Check sheet for the modelled part. Datum: model origin and axes. Units: mm. Coordinates: 2 decimals unless noted, no trailing zeros. Write each loop counter-clockwise with the first axis right and the second up, starting at its lowest first coordinate (ties: lowest second). Pieces come first, ordered by that corner, then holes. Notation, with made-up numbers: (-20.5, 35.25) - (-12.5, 35.25) arc R16 cw to (-12.5, 64.25) - close; hole circle Ø1 at (69.25, 59.5). An arc over 180 degrees is marked (long way). Use one line per item in the form item = value. Start each with the question number.
1. Cross-section at B-B on z = 1.25. Record the boundary of the cut face in (x, y), then the cut area to 3 significant figures.
2. Cross-section at A-A on x = -47. Record the boundary of the cut face in (y, z), then the cut area to 3 significant figures.
3. Scan lines: line 1 along X through (y, z) = (275.75, 1.6); line 2 along X through (y, z) = (280.75, 0.7); line 3 along X through (y, z) = (269, 0.65). Record each from-to range of solid material in increasing order.
Autodesk Inventor part; units mm, degrees
ref_plane "YZ Plane" through (0, 0, 0) normal (1, 0, 0) x (0, 1, 0)
ref_plane "XZ Plane" through (0, 0, 0) normal (0, 1, 0) x (-1, 0, 0)
ref_plane "XY Plane" through (0, 0, 0) normal (0, 0, 1) x (1, 0, 0)
sketch "Sketch1" plane through (0, 0, 0) normal (0, 0, 1) x (1, 0, 0)
  arc A0 (-89.3851, 275.0837) -> (-93.3851, 275.0837) centre (-91.3851, 275.0837) ccw
  line L0 (-89.3851, 275.0837) -> (-89.3851, 230.0837)
  arc A1 (-93.3851, 230.0837) -> (-89.3851, 230.0837) centre (-91.3851, 230.0837) ccw
  line L1 (-93.3851, 230.0837) -> (-93.3851, 275.0837)
  arc A2 (-44.3851, 275.0837) -> (-48.3851, 275.0837) centre (-46.3851, 275.0837) ccw
  line L2 (-44.3851, 275.0837) -> (-44.3851, 230.0837)
  arc A3 (-48.3851, 230.0837) -> (-44.3851, 230.0837) centre (-46.3851, 230.0837) ccw
  line L3 (-48.3851, 230.0837) -> (-48.3851, 275.0837)
  circle A4 centre (-6.132, -79.3472) radius 1.25
  circle A5 centre (-145.3842, 185.8247) radius 1.5
  circle A6 centre (-153.8932, -1.3222) radius 1.5
  circle A7 centre (-145.3842, -79.3472) radius 1.5
  circle A8 centre (-129.8902, 6.8528) radius 1.5
  circle A9 centre (-116.3012, -71.1722) radius 1.5
  circle A10 centre (-129.8902, 272.0247) radius 1.5
  circle A11 centre (-129.8902, 185.8247) radius 1.5
  circle A12 centre (-116.3012, 263.8497) radius 1.5
  circle A13 centre (17.871, -71.1722) radius 1.5
  circle A14 centre (-6.132, 6.8528) radius 1.5
  circle A15 centre (-19.721, -1.3222) radius 1.5
  circle A16 centre (17.871, 263.8497) radius 1.5
  circle A17 centre (9.362, 272.0247) radius 1.5
  circle A18 centre (9.362, 185.8247) radius 1.5
  circle A19 centre (-19.721, 193.9997) radius 1.5
  circle A20 centre (-19.721, 263.8497) radius 1.5
  circle A21 centre (-6.132, 185.8247) radius 1.5
  circle A22 centre (-6.132, 272.0247) radius 1.5
  circle A23 centre (17.871, 193.9997) radius 1.5
  circle A24 centre (-19.721, -71.1722) radius 1.5
  circle A25 centre (9.362, -79.3472) radius 1.5
  circle A26 centre (9.362, 6.8528) radius 1.5
  circle A27 centre (17.871, -1.3222) radius 1.5
  circle A28 centre (-116.3012, 193.9997) radius 1.5
  circle A29 centre (-153.8932, 193.9997) radius 1.5
  circle A30 centre (-153.8932, 263.8497) radius 1.5
  circle A31 centre (-145.3842, 6.8528) radius 1.5
  circle A32 centre (-129.8902, -79.3472) radius 1.5
  circle A33 centre (-153.8932, -71.1722) radius 1.5
  circle A34 centre (-116.3012, -1.3222) radius 1.5
  circle A35 centre (-145.3842, 272.0247) radius 1.5
  arc A36 (81.2372, 206.8201) -> (56.4499, 266.1206) centre (-44.5185, 189.0856) ccw
  ellipse E0 centre (-68.0111, 96.3387) end of major axis (-68.0111, -141.4053) minor radius 177.8 (56.4499, 266.1206) -> (-192.4721, 266.1206) ccw
  arc A37 (-192.4721, 266.1206) -> (-217.2594, 206.8201) centre (-91.5037, 189.0856) ccw
  arc A38 (-217.2594, 206.8201) -> (-217.2594, -14.1426) centre (566.1677, 96.3387) ccw
  arc A39 (-217.2594, -14.1426) -> (-192.4721, -73.4431) centre (-91.5037, 3.5918) ccw
  ellipse E1 centre (-68.0111, 96.3387) end of major axis (-68.0111, -141.4053) minor radius 177.8 (-192.4721, -73.4431) -> (56.4499, -73.4431) ccw
  arc A40 (56.4499, -73.4431) -> (81.2372, -14.1426) centre (-44.5185, 3.5918) ccw
  arc A41 (81.2372, -14.1426) -> (81.2372, 206.8201) centre (-702.1899, 96.3387) ccw
  circle A42 centre (-36.4956, 248.9087) radius 1.25
  circle A43 centre (-101.2746, 318.7587) radius 1.25
  circle A44 centre (-101.2746, 248.9087) radius 1.25
  circle A45 centre (-36.4956, 318.7587) radius 1.25
  circle A46 centre (-77.2861, -128.5803) radius 1.25
  circle A47 centre (-92.2681, -54.079) radius 1.25
  circle A48 centre (-53.9141, -54.079) radius 1.25
  circle A49 centre (-58.7361, -128.5803) radius 1.25
  line L4 (-82.971, -17.5241) -> (-82.971, 43.3967)
  line L5 (-82.971, 43.3967) -> (-52.491, 43.3967)
  line L6 (-52.491, 43.3967) -> (-52.491, -17.5241)
  line L7 (-52.491, -17.5241) -> (-82.971, -17.5241)
  circle A50 centre (-68.0111, 137.616) radius 35
  line L8 (-123.7158, 171.3631) -> (-119.7158, 171.3631)
  arc A51 (-119.7158, 168.3632) -> (-119.7158, 171.3631) centre (-119.7158, 169.8631) ccw
  line L9 (-119.7158, 168.3632) -> (-123.7158, 168.3632)
  arc A52 (-123.7158, 171.3631) -> (-123.7158, 168.3632) centre (-123.7158, 169.8631) ccw
  line L10 (-123.6698, 106.6744) -> (-119.6698, 106.6744)
  arc A53 (-119.6698, 103.6746) -> (-119.6698, 106.6744) centre (-119.6698, 105.1745) ccw
  line L11 (-119.6698, 103.6746) -> (-123.6698, 103.6746)
  arc A54 (-123.6698, 106.6744) -> (-123.6698, 103.6746) centre (-123.6698, 105.1745) ccw
  line L12 (-9.1669, 171.4444) -> (-5.1669, 171.4444)
  arc A55 (-5.1669, 168.4446) -> (-5.1669, 171.4444) centre (-5.1669, 169.9445) ccw
  line L13 (-5.1669, 168.4446) -> (-9.1669, 168.4446)
  arc A56 (-9.1669, 171.4444) -> (-9.1669, 168.4446) centre (-9.1669, 169.9445) ccw
  line L14 (-5.1669, 103.6742) -> (-9.1669, 103.6742)
  arc A57 (-9.1669, 106.6741) -> (-9.1669, 103.6742) centre (-9.1669, 105.1742) ccw
  line L15 (-9.1669, 106.6741) -> (-5.1669, 106.6741)
  arc A58 (-5.1669, 103.6742) -> (-5.1669, 106.6741) centre (-5.1669, 105.1742) ccw
  arc A59 (-34.0816, 86.6493) -> (-37.0792, 86.6494) centre (-35.5804, 86.6492) ccw
  line L16 (-34.0816, 86.6493) -> (-34.0814, 82.6493)
  arc A60 (-37.0794, 82.6493) -> (-34.0814, 82.6493) centre (-35.5804, 82.6492) ccw
  line L17 (-37.0794, 82.6493) -> (-37.0792, 86.6494)
  arc A61 (-34.0865, 201.0395) -> (-37.0841, 201.0395) centre (-35.5853, 201.0395) ccw
  line L18 (-34.0865, 201.0395) -> (-34.0863, 197.0396)
  arc A62 (-37.0843, 197.0395) -> (-34.0863, 197.0396) centre (-35.5853, 197.0395) ccw
  line L19 (-37.0843, 197.0395) -> (-37.0841, 201.0395)
  arc A63 (-34.0812, 78.9993) -> (-37.0788, 78.9992) centre (-35.58, 78.9992) ccw
  line L20 (-34.0812, 78.9993) -> (-34.081, 74.9993)
  arc A64 (-37.079, 74.9993) -> (-34.081, 74.9993) centre (-35.58, 74.9992) ccw
  line L21 (-37.079, 74.9993) -> (-37.0788, 78.9992)
  arc A65 (-98.9325, 193.3865) -> (-101.9301, 193.3866) centre (-100.4313, 193.3865) ccw
  line L22 (-98.9325, 193.3865) -> (-98.9323, 189.3866)
  arc A66 (-101.9303, 189.3866) -> (-98.9323, 189.3866) centre (-100.4313, 189.3865) ccw
  line L23 (-101.9303, 189.3866) -> (-101.9301, 193.3866)
  circle A67 centre (-95.163, -4.4165) radius 1.25
  circle A68 centre (-36.616, 37.0467) radius 1.25
  circle A69 centre (-46.141, -14.3491) radius 1.25
  circle A70 centre (-36.616, -11.1741) radius 1.25
  circle A71 centre (-36.616, 12.9421) radius 1.25
  circle A72 centre (-46.141, 40.2217) radius 1.25
  circle A73 centre (-95.163, 40.4375) radius 1.25
  arc A74 (-98.8512, 78.9533) -> (-101.8488, 78.9533) centre (-100.35, 78.9533) ccw
  line L24 (-98.8512, 78.9533) -> (-98.851, 74.9533)
  arc A75 (-101.849, 74.9533) -> (-98.851, 74.9533) centre (-100.35, 74.9533) ccw
  line L25 (-101.849, 74.9533) -> (-101.8488, 78.9533)
  line L26 (-34.0865, 193.3895) -> (-34.0863, 189.3896)
  arc A76 (-37.0843, 189.3896) -> (-34.0863, 189.3896) centre (-35.5853, 189.3895) ccw
  line L27 (-37.0843, 189.3896) -> (-37.0841, 193.3896)
  arc A77 (-34.0865, 193.3895) -> (-37.0841, 193.3896) centre (-35.5853, 193.3895) ccw
  arc A78 (-98.9379, 201.0395) -> (-101.9362, 200.9947) centre (-100.4367, 200.9934) ccw
  line L28 (-98.9379, 201.0395) -> (-98.9377, 196.9935)
  arc A79 (-101.9357, 196.9932) -> (-98.9377, 196.9935) centre (-100.4367, 196.9934) ccw
  line L29 (-101.9357, 196.9932) -> (-101.9362, 200.9947)
  arc A80 (-98.8567, 86.6032) -> (-101.8543, 86.6033) centre (-100.3555, 86.6032) ccw
  line L30 (-98.8567, 86.6032) -> (-98.8565, 82.6033)
  arc A81 (-101.8544, 82.6033) -> (-98.8565, 82.6033) centre (-100.3555, 82.6032) ccw
  line L31 (-101.8544, 82.6033) -> (-101.8543, 86.6033)
  line L32 (-16.8169, 106.6744) -> (-12.8169, 106.6744)
  arc A82 (-12.8169, 103.6746) -> (-12.8169, 106.6744) centre (-12.8169, 105.1745) ccw
  line L33 (-12.8169, 103.6746) -> (-16.8169, 103.6746)
  arc A83 (-16.8169, 106.6744) -> (-16.8169, 103.6746) centre (-16.8169, 105.1745) ccw
  line L34 (-16.8629, 171.439) -> (-12.8629, 171.439)
  arc A84 (-12.8629, 168.4391) -> (-12.8629, 171.439) centre (-12.8629, 169.9391) ccw
  line L35 (-12.8629, 168.4391) -> (-16.8629, 168.4391)
  arc A85 (-16.8629, 171.439) -> (-16.8629, 168.4391) centre (-16.8629, 169.9391) ccw
  line L36 (-131.3198, 106.6744) -> (-127.3198, 106.6744)
  arc A86 (-127.3198, 103.6746) -> (-127.3198, 106.6744) centre (-127.3198, 105.1745) ccw
  line L37 (-127.3198, 103.6746) -> (-131.3198, 103.6746)
  arc A87 (-131.3198, 106.6744) -> (-131.3198, 103.6746) centre (-131.3198, 105.1745) ccw
  line L38 (-131.3658, 171.3576) -> (-127.3658, 171.3576)
  arc A88 (-127.3658, 168.3578) -> (-127.3658, 171.3576) centre (-127.3658, 169.8577) ccw
  line L39 (-127.3658, 168.3578) -> (-131.3658, 168.3578)
  arc A89 (-131.3658, 171.3576) -> (-131.3658, 168.3578) centre (-131.3658, 169.8577) ccw
  circle A90 centre (-46.3851, 275.0837) radius 1.25
  circle A91 centre (-91.3851, 275.0837) radius 1.25
  line L40 (-41.3851, 222.0837) -> (-41.3851, 377.0837)
  line L41 (-96.3851, 377.0837) -> (-96.3851, 222.0837)
  line L42 (-46.3851, 275.0837) -> (-41.3851, 275.0837)
  line L43 (-41.3851, 275.0837) -> (-41.3851, 268.0837)
  line L44 (-41.3851, 268.0837) -> (-41.3851, 282.0837)
  line L45 (-41.3851, 282.0837) -> (-96.3851, 282.0837)
  line L46 (-41.3851, 274.0837) -> (-41.3851, 282.0837)
  line L47 (-41.3851, 282.0837) -> (-96.3851, 282.0837)
  line L48 (-96.3851, 282.0837) -> (-96.3851, 270.0837)
  line L49 (-41.3851, 270.0837) -> (-41.3851, 282.0837)
  line L50 (-41.3851, 282.0837) -> (-96.3851, 282.0837)
  line L51 (-96.3851, 282.0837) -> (-96.3851, 268.0837)
  line L52 (-96.3851, 268.0837) -> (-41.3851, 268.0837)
  line L53 (-41.3851, 268.0837) -> (-41.3851, 282.0837)
  point P0 (0, 0)
  dimension "d0" = 7
  dimension "d1" = 14
extrude "Extrusion1" add sketch "Sketch1" along normal blind 3 contours L0 L52 L1 A0 | A0 L1 L52 L41 L45 L40 L42 A2 L3 L0 | L3 A2 L2 L52 | L2 L42 L40 L52
fillet "Fillet1" radius 2 4 edges at (-96.3851, 282.0837, 1.5) (-96.3851, 268.0837, 1.5) (-41.3851, 268.0837, 1.5) (-41.3851, 282.0837, 1.5)
properties part number "HeadSlide"
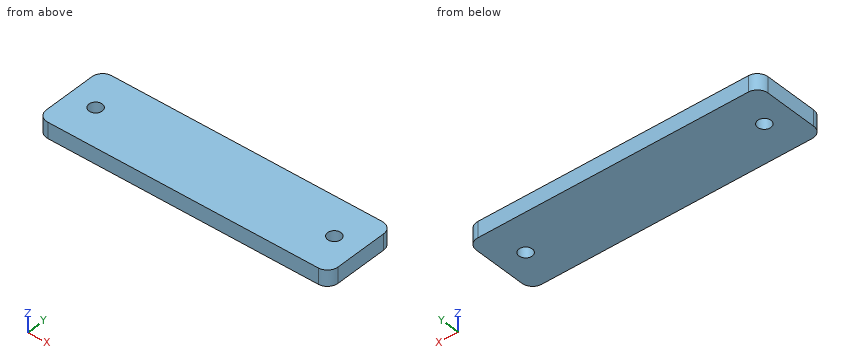
Final values:
q1.outline = (-96.39, 270.08) arc R2 ccw to (-94.39, 268.08) - (-43.39, 268.08) arc R2 ccw to (-41.39, 270.08) - (-41.39, 280.08) arc R2 ccw to (-43.39, 282.08) - (-94.39, 282.08) arc R2 ccw to (-96.39, 280.08) - close; hole circle Ø2.5 at (-91.39, 275.08); hole circle Ø2.5 at (-46.39, 275.08)
q1.area = 757 mm²
q2.outline = (268.08, 0) - (274, 0) - (274, 3) - (268.08, 3) - close; (276.17, 0) - (282.08, 0) - (282.08, 3) - (276.17, 3) - close
q2.area = 35.5 mm²
q3.line_1 = -96.39 to -92.44, -90.33 to -47.44, -45.33 to -41.39
q3.line_2 = -96.27 to -41.5
q3.line_3 = -96.07 to -41.7
